Verification items for the finished model (mm, model axes). A direction names the side the tool comes from. Round coordinates to 2 decimals unless told otherwise and drop trailing zeros. Write each loop counter-clockwise with the first axis right and the second up, starting at its lowest first coordinate (ties: lowest second). Pieces come first, ordered by that corner, then holes.
from build123d import *

# Parameters (mm, degrees)
F0_W      = 36
F0_H      = 24
F1_DEPTH  = 21.5
F2_R      = 1.7
F3_DEPTH  = 36.001
F5_DEPTH  = 4
F6_R      = 3.25
F7_DEPTH  = 6.5
F8_R      = 1.5
F9_DEPTH  = 6
F10_W     = 2
F10_H     = 22
F10_R     = 1.75
F11_DEPTH = 26.001
F12_R     = 3.5
F13_DEPTH = 15
F14_R     = 1.5
F15_DEPTH = 6
F16_R     = 1.5
F17_DEPTH = 6


with BuildPart() as f1:
    # F0 (on Front) → F1 (new body)
    with BuildSketch(Plane.XZ):
        Rectangle(F0_W, F0_H)
    extrude(amount=F1_DEPTH)

    # F2 (on face) → F3 (cut, through all)
    with BuildSketch(Plane(origin=(-18, 0, 0), x_dir=(0, -1, 0), z_dir=(-1, 0, 0))):
        with Locations((15.5, 7.5)):
            Circle(F2_R)
        with Locations((5.5, -7.5)):
            Circle(F2_R)
        with Locations((5.5, 7.5)):
            Circle(F2_R)
        with Locations((15.5, -7.5)):
            Circle(F2_R)
    extrude(amount=-F3_DEPTH, mode=Mode.SUBTRACT)

    # F4 (on face) → F5 (join)
    with BuildSketch(Plane(origin=(-18, 0, 0), x_dir=(0, -1, 0), z_dir=(-1, 0, 0))):
        Polygon((0, -4), (0, 4), (-4.5, 4), (-4.5, 1.127949), (-3.5, 0.86), (-2.3, 0.86), (-2.3, -0.86), (-3.5, -0.86), (-4.5, -1.127949), (-4.5, -4), align=None)
    extrude(amount=-F5_DEPTH)

    # F6 (on face) → F7 (cut)
    with BuildSketch(Plane(origin=(-18, 0, 0), x_dir=(0, -1, 0), z_dir=(-1, 0, 0))):
        with Locations((15.5, 7.5)):
            Circle(F6_R)
        with Locations((5.5, 7.5)):
            Circle(F6_R)
        with Locations((5.5, -7.5)):
            Circle(F6_R)
        with Locations((15.5, -7.5)):
            Circle(F6_R)
    extrude(amount=-F7_DEPTH, mode=Mode.SUBTRACT)

    # F8 (on face) → F9 (cut)
    with BuildSketch(Plane.XZ.offset(21.5)):
        with Locations((-12, 0)):
            Circle(F8_R)
        with Locations((2, 0)):
            Circle(F8_R)
    extrude(amount=-F9_DEPTH, mode=Mode.SUBTRACT)

    # F10 (on face) → F11 (cut, through all)
    with BuildSketch(Plane.XZ.offset(21.5)):
        with Locations((17, 1)):
            Rectangle(F10_W, F10_H)
        with Locations((-5, 0)):
            Circle(F10_R)
    extrude(amount=-F11_DEPTH, mode=Mode.SUBTRACT)

    # F12 (on face) → F13 (cut)
    with BuildSketch(Plane.XZ.offset(21.5)):
        with Locations((-5, 0)):
            Circle(F12_R)
    extrude(amount=-F13_DEPTH, mode=Mode.SUBTRACT)

    # F14 (on face) → F15 (cut)
    with BuildSketch(Plane(origin=(0, 0, -12), x_dir=(1, 0, 0), z_dir=(0, 0, -1))):
        with Locations((12, 9.5)):
            Circle(F14_R)
    extrude(amount=-F15_DEPTH, mode=Mode.SUBTRACT)

    # F16 (on face) → F17 (cut)
    with BuildSketch(Plane(origin=(0, 0, 0), x_dir=(-1, 0, 0), z_dir=(0, 1, 0))):
        with Locations((-12, 0)):
            Circle(F16_R)
    extrude(amount=-F17_DEPTH, mode=Mode.SUBTRACT)


solid = f1.part
Q1. Sectioned sample at C-C (x = 12). Enter the section's corners in (y, z), plus the area to 3 significant figures.
Recorded:
outline: (-21.5, -12) - (-11, -12) - (-11, -6) - (-8, -6) - (-8, -12) - (0, -12) - (0, -1.5) - (-6, -1.5) - (-6, 1.5) - (0, 1.5) - (0, 12) - (-21.5, 12) - close; hole circle Ø3.4 at (-15.5, -7.5); hole circle Ø3.4 at (-15.5, 7.5); hole circle Ø3.4 at (-5.5, -7.5); hole circle Ø3.4 at (-5.5, 7.5)
area: 444 mm2
Q2. Release check for a two-part mould opening along Z. For faces 1 (the flat face through (-11.5, -17, -9)), 2 (the flat face through (0, -11, -12)), 3 (the flat face through (-16, 3, -0.86)), 4 (the flat face through (-1, -11, 12)) record: released by +Z, released by -Z, zero draft, split by the parting line, or undercut.
Recorded:
face 1: undercut
face 2: released by -Z
face 3: undercut
face 4: released by +Z
Q3. Tool access check on faces 5 (the flat face through (12, -10, -6)), 6 (the flat face through (2, -15.5, 0)), 7 (the flat face through (17, -11, -10)). Record the directions out of +Z, -Z, +X, -X, +Y, -Y that give a thin tool (end or side, any length) a straight path to the whole face; none if there is none.
Recorded:
face 5: -Z
face 6: -Y
face 7: +Z, +X, +Y, -Y
Q4. Sectioned sample at D-D (z = 7.5). Enter the section's corners in (x, y).
Recorded:
outline: (-18, -21.5) - (16, -21.5) - (16, -17.2) - (-11.5, -17.2) - (-11.5, -18.75) - (-18, -18.75) - close; (-18, -12.25) - (-11.5, -12.25) - (-11.5, -13.8) - (16, -13.8) - (16, -7.2) - (-11.5, -7.2) - (-11.5, -8.75) - (-18, -8.75) - close; (-18, -2.25) - (-11.5, -2.25) - (-11.5, -3.8) - (16, -3.8) - (16, 0) - (-18, 0) - close
Q5. Depth check by flat-ended pin: P1, Ø4, axis at x = -6, z = 7.5, coming from the +Y side; P2, Ø11, axis at y = -6.5, z = 1, coming from the +X side; P3, Ø5.5, axis at x = -5, z = 0, coming from the -Y side. Enter the tip coordinate at first touch or a pass-through.
Recorded:
P1: stops at y = 0
P2: stops at x = 16
P3: stops at y = -6.5
Q6. Sectioned sample at A-A (z = -7.5). Enter the section's corners in (x, y).
Recorded:
outline: (-18, -21.5) - (16, -21.5) - (16, -17.2) - (-11.5, -17.2) - (-11.5, -18.75) - (-18, -18.75) - close; (-18, -12.25) - (-11.5, -12.25) - (-11.5, -13.8) - (16, -13.8) - (16, -7.2) - (-11.5, -7.2) - (-11.5, -8.75) - (-18, -8.75) - close; (-18, -2.25) - (-11.5, -2.25) - (-11.5, -3.8) - (16, -3.8) - (16, 0) - (-18, 0) - close; hole circle Ø3 at (12, -9.5)
Q7. Material ranges on line 1 along Z through (x, y) = (8.25, -15.5); line 2 along Z through (x, y) = (-14, -5.5); line 3 along Y through (x, z) = (12, -10.45), recorded low to high.
Recorded:
line 1: z = -12 to -9.2, -5.8 to 5.8, 9.2 to 12
line 2: z = -12 to -10.75, -4.25 to 4.25, 10.75 to 12
line 3: y = -21.5 to -11, -8 to 0
Q8. Sectioned sample at B-B (z = 0). Enter the section's corners in (x, y).
Recorded:
outline: (-18, -21.5) - (-13.5, -21.5) - (-13.5, -15.5) - (-10.5, -15.5) - (-10.5, -21.5) - (-8.5, -21.5) - (-8.5, -6.5) - (-6.75, -6.5) - (-6.75, 0) - (-14, 0) - (-14, 2.3) - (-18, 2.3) - close; (-3.25, -6.5) - (-1.5, -6.5) - (-1.5, -21.5) - (0.5, -21.5) - (0.5, -15.5) - (3.5, -15.5) - (3.5, -21.5) - (16, -21.5) - (16, 0) - (13.5, 0) - (13.5, -6) - (10.5, -6) - (10.5, 0) - (-3.25, 0) - close
